```python
from build123d import *

# Parameters (mm, degrees)
BASE_EXTRUDE_DEPTH = 12.7
CHAMFER3_SIZE      = 2.54


with BuildPart() as part:
    # Sketch1 → Base-Extrude (new body)
    with BuildSketch(Plane.XY):
        Polygon((0, 0), (152.4, 0), (152.4, 19.05), (25.4, 241.3), (0, 241.3), align=None)
        with BuildLine():
            Line((15.24, 21.59), (15.24, 204.451463804))
            ThreePointArc((15.24, 204.451463804), (19.960158612, 210.588736573), (27.103343952, 207.601946062))
            Line((27.103343952, 207.601946062), (131.595608983, 24.740482259))
            ThreePointArc((131.595608983, 24.740482259), (131.574444122, 18.402764704), (126.082265031, 15.24))
            Line((126.082265031, 15.24), (21.59, 15.24))
            ThreePointArc((21.59, 15.24), (17.099871939, 17.099871939), (15.24, 21.59))
        make_face(mode=Mode.SUBTRACT)
    extrude(amount=BASE_EXTRUDE_DEPTH)

    # Chamfer3
    chamfer3_edges = [part.edges().sort_by_distance(p)[0] for p in [
        (76.2, 0, 0),
    ]]
    chamfer(chamfer3_edges, length=CHAMFER3_SIZE)


solid = part.part
```
The listing builds one solid part. Answer for the finished solid, in the listing's coordinates (mm). A direction names the side the tool comes from. Round coordinates to 2 decimals unless told otherwise and drop trailing zeros. Loops run counter-clockwise (first coordinate to the right, second up) from the corner with the lowest first, then second, coordinate; pieces in that order, holes last.
1) Consider line 1 (Y direction, x = 22, z = 11.25); line 2 (X direction, y = 137, z = 11.75); line 3 (Y direction, x = 22.5, z = 6.75). Determine where each line is inside the solid, lowest interval first.
Outcome:
line 1: y = 0 to 15.24, 210.79 to 241.3
line 2: x = 0 to 15.24, 67.45 to 85
line 3: y = 0 to 15.24, 210.74 to 241.3
2) A cutting plane is placed at A-A on z = 7.5. Determine the outline of the cut face in (x, y), plus the area to 3 significant figures.
Outcome:
outline: (0, 0) - (152.4, 0) - (152.4, 19.05) - (25.4, 241.3) - (0, 241.3) - close; hole (15.24, 21.59) arc R6.35 ccw to (21.59, 15.24) - (126.08, 15.24) arc R6.35 ccw to (131.6, 24.74) - (27.1, 207.6) arc R6.35 ccw to (15.24, 204.45) - close
area: 9,820 mm2
3) Given P1, Ø6.5, axis at y = 89, z = 8, coming from the +X side; P2, Ø4, axis at x = 88, z = 7.5, coming from the +Y side; P3, Ø4, axis at x = 83.5, z = 5.5, coming from the +Y side (3 decimals), each flat-ended and moving along its own axis, determine where each tip first touches the part or whether it passes through.
Outcome:
P1: stops at x = 114.29
P2: stops at y = 135.25
P3: stops at y = 143.125
4) A cutting plane is placed at C-C on y = 138.5. Determine the outline of the cut face in (x, z), plus the area to 3 significant figures.
Outcome:
outline: (0, 0) - (15.24, 0) - (15.24, 12.7) - (0, 12.7) - close; (66.59, 0) - (84.14, 0) - (84.14, 12.7) - (66.59, 12.7) - close
area: 416 mm2
5) For a pull along Y with two mould halves and no side action, classify faces 3 (the face through (152.4, 9, 6)), 4 (the face through (17.1, 17.1, 6.3)), 5 (the face through (75, 0, 8)) as released by +Y, released by -Y, zero draft, split by the parting line, or undercut.
Outcome:
face 3: zero draft
face 4: undercut
face 5: released by -Y
6) A cutting plane is placed at B-B on x = 105.5. Determine the outline of the cut face in (y, z) (3 decimals), plus the area to 3 significant figures.
Outcome:
outline: (0, 2.54) - (2.54, 0) - (15.24, 0) - (15.24, 12.7) - (0, 12.7) - close; (70.408, 0) - (101.125, 0) - (101.125, 12.7) - (70.408, 12.7) - close
area: 580 mm2
7) For faces 1 (the face through (78.62, 117.45, 6.26)), 2 (the face through (81, 114, 0)), determine the directions among +Z, -Z, +X, -X, +Y, -Y from which every point of the face is accessible in a straight line to the end or side of a thin tool.
Outcome:
face 1: +Z, -Z
face 2: -Z, +X, -X, +Y, -Y
